Verification items for the finished model (mm, model axes). A direction names the side the tool comes from. Round coordinates to 2 decimals unless told otherwise and drop trailing zeros. Loops run counter-clockwise (first coordinate to the right, second up) from the corner with the lowest first, then second, coordinate; pieces in that order, holes last. Notation, with made-up numbers: M 64.5,76 L 73.5,76 A22 cw 73.5,92 Z; hole C 12,-7.75 d6. An arc over 180 degrees is marked long. One line per item, written item: value.
from build123d import *

# Parameters (mm, degrees)
SKETCH1_R           = 2.2479
SKETCH1_R_2         = 2.2
EXTRUDE_BODY_DEPTH  = 4
SKETCH5_W           = 10
SKETCH5_H           = 10
SKETCH5_R           = 2.2
SKETCH5_R_2         = 2.2479
EXTRUDE_LEGS_DEPTH  = 10
SKETCH6_W           = 45
SKETCH6_H           = 0.5
BOSS_EXTRUDE1_DEPTH = 4
CUT_EXTRUDE1_DEPTH  = 45


with BuildPart() as part:
    # Sketch1 → Extrude-Body (new body)
    with BuildSketch(Plane(origin=(0, 0, 0), x_dir=(1, 0, 0), z_dir=(0, 1, 0))):
        with BuildLine():
            Line((10, -10), (10, 10))
            Line((10, 10), (45, 10))
            Line((45, 10), (55, 10))
            Line((55, 10), (55, 20))
            Line((55, 20), (55, 32))
            Line((55, 32), (45, 32))
            ThreePointArc((45, 32), (27.5, 15), (10, 32))
            Line((10, 32), (0, 32))
            Line((0, 32), (0, 20))
            Line((0, 20), (0, -20))
            Line((0, -20), (0, -32))
            Line((0, -32), (10, -32))
            ThreePointArc((10, -32), (27.5, -15), (45, -32))
            Line((45, -32), (55, -32))
            Line((55, -32), (55, -20))
            Line((55, -20), (55, -10))
            Line((55, -10), (45, -10))
            Line((45, -10), (10, -10))
        make_face()
        with Locations(Location((4.755333622, -26.250570114, 0), (0, 0, 270))):
            Circle(SKETCH1_R, mode=Mode.SUBTRACT)
        with Locations(Location((50, -27, 0), (0, 0, 270))):
            Circle(SKETCH1_R_2, mode=Mode.SUBTRACT)
        with Locations(Location((5.244634233, 26.247149693, 0), (0, 0, 270))):
            Circle(SKETCH1_R, mode=Mode.SUBTRACT)
        with Locations(Location((50, 27, 0), (0, 0, 270))):
            Circle(SKETCH1_R_2, mode=Mode.SUBTRACT)
    extrude(amount=EXTRUDE_BODY_DEPTH)

    # Sketch5 → Extrude-Legs (add)
    # profile 1 of 4: a face of its own
    with BuildSketch(Plane(origin=(0, 4, 0), x_dir=(1, 0, 0), z_dir=(0, 1, 0))):
        with Locations((50, -27)):
            Rectangle(SKETCH5_W, SKETCH5_H)
        with Locations(Location((50, -27, 0), (0, 0, 270))):
            Circle(SKETCH5_R, mode=Mode.SUBTRACT)
    # profile 2 of 4: a face of its own
    with BuildSketch(Plane(origin=(0, 4, 0), x_dir=(1, 0, 0), z_dir=(0, 1, 0))):
        with Locations((50, 27)):
            Rectangle(SKETCH5_W, SKETCH5_H)
        with Locations(Location((50, 27, 0), (0, 0, 270))):
            Circle(SKETCH5_R, mode=Mode.SUBTRACT)
    # profile 3 of 4: a face of its own
    with BuildSketch(Plane(origin=(0, 4, 0), x_dir=(1, 0, 0), z_dir=(0, 1, 0))):
        with Locations((5, 27)):
            Rectangle(SKETCH5_W, SKETCH5_H)
        with Locations(Location((5.244634233, 26.247149693, 0), (0, 0, 270))):
            Circle(SKETCH5_R_2, mode=Mode.SUBTRACT)
    # profile 4 of 4: a face of its own
    with BuildSketch(Plane(origin=(0, 4, 0), x_dir=(1, 0, 0), z_dir=(0, 1, 0))):
        with Locations((5, -27)):
            Rectangle(SKETCH5_W, SKETCH5_H)
        with Locations(Location((4.755333622, -26.250570114, 0), (0, 0, 270))):
            Circle(SKETCH5_R_2, mode=Mode.SUBTRACT)
    extrude(amount=EXTRUDE_LEGS_DEPTH)

    # Sketch6 → Boss-Extrude1 (add)
    with BuildSketch(Plane(origin=(0, 4, 0), x_dir=(1, 0, 0), z_dir=(0, 1, 0))):
        with Locations((32.5, -9.75)):
            Rectangle(SKETCH6_W, SKETCH6_H)
        with Locations((32.5, 9.75)):
            Rectangle(SKETCH6_W, SKETCH6_H)
    extrude(amount=-BOSS_EXTRUDE1_DEPTH)

    # Sketch7 → Cut-Extrude1 (cut)
    with BuildSketch(Plane(origin=(55, 0, 0), x_dir=(0, 0, -1), z_dir=(1, 0, 0))):
        with BuildLine():
            Line((-10.207106781, 2.707106781), (-11.5, 4))
            Line((-11.5, 4), (-9.5, 4))
            Line((-9.5, 4), (-9.5, 0))
            Line((-9.5, 0), (-11.5, 0))
            Line((-11.5, 0), (-10.207106781, 1.292893219))
            ThreePointArc((-10.207106781, 1.292893219), (-9.914213562, 2), (-10.207106781, 2.707106781))
        make_face()
        with BuildLine():
            Line((10.207106781, 2.707106781), (11.5, 4))
            Line((11.5, 4), (9.5, 4))
            Line((9.5, 4), (9.5, 0))
            Line((9.5, 0), (11.5, 0))
            Line((11.5, 0), (10.207106781, 1.292893219))
            ThreePointArc((10.207106781, 1.292893219), (9.914213562, 2), (10.207106781, 2.707106781))
        make_face()
    extrude(amount=-CUT_EXTRUDE1_DEPTH, mode=Mode.SUBTRACT)


solid = part.part
(1) Sectioned sample at C-C on z = 27. Enter the section's corners in (x, y).
Completed:
outline: M 0,0 L 2.64,0 L 2.64,14 L 0,14 Z; M 6.87,0 L 10.88,0 L 10.88,4 L 10,4 L 10,14 L 6.87,14 Z; M 44.12,0 L 47.8,0 L 47.8,14 L 45,14 L 45,4 L 44.12,4 Z; M 52.2,0 L 55,0 L 55,14 L 52.2,14 Z
(2) Depth check by flat-ended pin: pin 1 Ø5 at (y, z) = (8.5, -28.5) entering from -X; pin 2 Ø2 at (x, y) = (16.5, 6.5) entering from -Z; pin 3 Ø1.2 at (y, z) = (3, -4.5) entering from +X. Enter the tip coordinate at first touch or a pass-through.
Completed:
pin 1: stops at x = 0
pin 2: passes through
pin 3: stops at x = 10
(3) Mould release check, pull along Z, two halves, no side actions. Record for faces 1 (the face through (10, 9, 27)), 2 (the face through (47.852, 6.902, -27.477)), 3 (the face through (27.878, 1.972, -15.004)): +Z half, -Z half, draft (parallel to the pull), parting line (faces both ways), or undercut.
Completed:
face 1: draft
face 2: undercut
face 3: -Z half
(4) Sectioned sample at D-D on x = 19. Enter the section's corners in (y, z).
Completed:
outline: M 0,-17.2 L 4,-17.2 L 4,-11.5 L 2.71,-10.21 A1 ccw 1.29,-10.21 L 0,-11.5 Z; M 0,11.5 L 1.29,10.21 A1 ccw 2.71,10.21 L 4,11.5 L 4,17.2 L 0,17.2 Z
(5) Sectioned sample at A-A on x = 50. Enter the section's corners in (y, z).
Completed:
outline: M 0,-32 L 14,-32 L 14,-29.2 L 0,-29.2 Z; M 0,-24.8 L 14,-24.8 L 14,-22 L 4,-22 L 4,-11.5 L 2.71,-10.21 A1 ccw 1.29,-10.21 L 0,-11.5 Z; M 0,11.5 L 1.29,10.21 A1 ccw 2.71,10.21 L 4,11.5 L 4,22 L 14,22 L 14,24.8 L 0,24.8 Z; M 0,29.2 L 14,29.2 L 14,32 L 0,32 Z
(6) Thickness scan on L1, parallel to X at y = 9, z = -27; L2, parallel to Y at x = 13, z = -17.5; L3, parallel to X at y = 3.25, z = -9. Record the ranges inside material, lowest first. Write a range as from..to.
Completed:
L1: x = 0..3.13, 7.36..10, 45..47.8, 52.2..55
L2: y = 0..4
L3: x = 0..10
(7) Tool access check on faces 4 (the face through (50, 9, 22)), 5 (the face through (45, 9, 27)), 6 (the face through (32.8, 0.6, -10.9)). Record the directions out of +Z, -Z, +X, -X, +Y, -Y that give a thin tool (end or side, any length) a straight path to the whole face; none if there is none.
Completed:
face 4: +X, -X, +Y
face 5: +Z, -Z, +Y
face 6: +X, -Y
(8) Sectioned sample at B-B on y = 10.25. Enter the section's corners in (x, z).
Completed:
outline: M 0,-32 L 10,-32 L 10,-22 L 0,-22 Z; M 0,22 L 10,22 L 10,32 L 0,32 Z; M 45,-32 L 55,-32 L 55,-22 L 45,-22 Z; M 45,22 L 55,22 L 55,32 L 45,32 Z; hole C 4.76,26.25 d4.5; hole C 5.24,-26.25 d4.5; hole C 50,-27 d4.4; hole C 50,27 d4.4
